```python
from build123d import *

# Parameters (mm, degrees)
F0_R     = 21.5
F0_R_2   = 19.2
F1_DEPTH = 40
F2_R     = 30
F2_R_2   = 12.5
F3_DEPTH = 5
F5_D     = 5
F6_SIZE  = 0.5


with BuildPart() as f1:
    # F0 (on Top) → F1 (new body)
    with BuildSketch(Plane.XY):
        Circle(F0_R)
        Circle(F0_R_2, mode=Mode.SUBTRACT)
    extrude(amount=F1_DEPTH)

    # F2 (on Top) → F3 (join)
    with BuildSketch(Plane.XY):
        Circle(F2_R)
        Circle(F2_R_2, mode=Mode.SUBTRACT)
    extrude(amount=-F3_DEPTH)

    # F5 (through all)
    with Locations(Plane(origin=(0, 0, -5), x_dir=(1, 0, 0), z_dir=(0, 0, -1))):
        with Locations((-24.75, 0), (0, 24.75), (24.75, 0), (0, -24.75)):
            Hole(F5_D / 2)

    # F6
    f6_edges = [f1.edges().sort_by_distance(p)[0] for p in [
        (-19.2, 0, 40),
    ]]
    chamfer(f6_edges, length=F6_SIZE)


solid = f1.part
```
The model under review builds one solid part; all positions refer to its coordinate system, in mm. A direction names the side the tool comes from. Coordinates: 2 decimals unless noted, no trailing zeros. Write each loop counter-clockwise with the first axis right and the second up, starting at its lowest first coordinate (ties: lowest second). Pieces come first, ordered by that corner, then holes.
1) The part is to be moulded in two halves that separate along Y. For faces 1 (the face through (-29.97, 1.32, -2.46)), 2 (the face through (19, -6, 40)), 3 (the face through (27.248, -0.11, -2.465)), say which applies: pulls with the +Y half, pulls with the -Y half, needs draft (parallel to the pull), parting line crosses it, or undercut.
2) Clearance check with flat-ended pins moving along their axes: pin 1 Ø1.5 at (x, z) = (7, 30) entering from -Y; pin 2 Ø3 at (x, y) = (-16.5, 23.5) entering from +Z; pin 3 Ø4 at (x, z) = (18, 6.5) entering from -Y. State where each tip first meets the part, or that it passes through.
3) Machinability: for faces 4 (the face through (0, -13, 0)), 5 (the face through (0.33, -27.23, -2.47)), which of the approach directions +Z, -Z, +X, -X, +Y, -Y give a long, thin tool a straight path to every point of the face, cutting with its end or side? Answer none if there is none.
4) We need section D-D on z = 14.5. State the section outline as (x, y) points, then the cut area to 3 significant figures.
5) We need section B-B on x = -24.75. State the section outline as (y, z) points, then the cut area to 3 significant figures.
6) To check wall thickness, follow probe 1 along Y at (x, z) = (0, -3.75); probe 2 along Z at (x, y) = (-11, -9); probe 3 along Y at (x, z) = (0, 10). State the ranges of each line that lie inside material, in increasing order.
7) We need section A-A on x = 0. State the section outline as (y, z) points.
Answer list:
1. face 1: parting line crosses it
1. face 2: needs draft
1. face 3: undercut
2. pin 1: stops at y = -20.57
2. pin 2: stops at z = 0
2. pin 3: stops at y = -14.36
3. face 4: +Z
3. face 5: +Z, -Z
4. outline: circle Ø43 at (0, 0); hole circle Ø38.4 at (0, 0)
4. area: 294 mm2
5. outline: (-16.95, -5) - (-2.5, -5) - (-2.5, 0) - (-16.95, 0) - close; (2.5, -5) - (16.95, -5) - (16.95, 0) - (2.5, 0) - close
5. area: 145 mm2
6. probe 1: y = -30 to -27.25, -22.25 to -12.5, 12.5 to 22.25, 27.25 to 30
6. probe 2: z = -5 to 0
6. probe 3: y = -21.5 to -19.2, 19.2 to 21.5
7. outline: (-30, -5) - (-27.25, -5) - (-27.25, 0) - (-30, 0) - close; (-22.25, -5) - (-12.5, -5) - (-12.5, 0) - (-19.2, 0) - (-19.2, 39.5) - (-19.7, 40) - (-21.5, 40) - (-21.5, 0) - (-22.25, 0) - close; (12.5, -5) - (22.25, -5) - (22.25, 0) - (21.5, 0) - (21.5, 40) - (19.7, 40) - (19.2, 39.5) - (19.2, 0) - (12.5, 0) - close; (27.25, -5) - (30, -5) - (30, 0) - (27.25, 0) - close
